Source: CAD feature listing. Evaluate the final solid. Frame: model axes, mm. A direction names the side the tool comes from. Round coordinates to 2 decimals unless told otherwise and drop trailing zeros. Order: outer loops, then holes, each group sorted by start corner. A loop starts at its lowest first (then second) coordinate and runs counter-clockwise, first axis right, second up. Notation, with made-up numbers: M -4,0.25 L 20,0.25 A28 ccw 20,28.25 Z; hole C 82.5,-3.5 d4. An arc over 180 degrees is marked long. Use one line per item in the form item = value. Start each with the question number.
Q1. Material intervals for probe 1 along X at (y, z) = (2.1, 39); probe 2 along Z at (x, y) = (1, 2.95); probe 3 along X at (y, z) = (1.6, -55), sorted ascending.
Q2. Pull-direction query (Z, two-part tool) for faces 1 (the conical face through (-41.21, 2.92, 39.85)), 2 (the conical face through (-41.21, 2.92, -37.93)), 3 (the flat face through (34, 5, -44)); classes: pulls with the +Z half, pulls with the -Z half, needs draft (parallel to the pull), parting line crosses it, or undercut.
Q3. Section A-A (z = -26). Return the cut outline in (x, y), plus the area to 3 significant figures.
Q4. Contact query for flat-ended pins moving along their axis: pin 1 (6 mm diameter, centred on x = -38.89, z = 38.89, fed in from +Y); pin 2 (5.5 mm diameter, centred on x = 55, z = 0, fed in from +Y). Output: stop coordinate, or through.
Q5. Section B-B (y = 1.3). Give the number of separate pieces and of enclosed holes in the cut face, plus the area to 3 significant figures.
Q6. Reachability of faces 4 (the flat face through (-39, 0, -1)), 5 (the cylindrical face through (-17.235, 4.507, 41.569)) from +Z, -Z, +X, -X, +Y, -Y: full face, straight path, thin tool, end or side. Return the list, or none.
from build123d import *

# Parameters (mm, degrees)
SKETCH1_W                                            = 327
SKETCH1_H                                            = 192
BOSS_EXTRUDE1_DEPTH                                  = 5
SKETCH2_R                                            = 35
CUT_EXTRUDE1_DEPTH                                   = 190.666154071
SKETCH3_R                                            = 45
CUT_EXTRUDE2_DEPTH                                   = 1
CSK_FOR_M4_HEX_SOCKET_COUNTERSUNK_HEAD_S_D           = 4.8
CSK_FOR_M4_HEX_SOCKET_COUNTERSUNK_HEAD_S_CSINK_D     = 9.18
CSK_FOR_M4_HEX_SOCKET_COUNTERSUNK_HEAD_S_CSINK_ANGLE = 90


with BuildPart() as part:
    # Sketch1 → Boss-Extrude1 (new body)
    with BuildSketch(Plane(origin=(0, 0, 0), x_dir=(1, 0, 0), z_dir=(0, 1, 0))):
        Rectangle(SKETCH1_W, SKETCH1_H)
    extrude(amount=BOSS_EXTRUDE1_DEPTH)

    # Sketch2 → Cut-Extrude1 (cut, through all)
    with BuildSketch(Plane(origin=(0, 5, 0), x_dir=(1, 0, 0), z_dir=(0, 1, 0))):
        with Locations(Location((0, 0, 0), (0, 0, 270))):
            Circle(SKETCH2_R)
    extrude(amount=-CUT_EXTRUDE1_DEPTH, mode=Mode.SUBTRACT)

    # Sketch3 → Cut-Extrude2 (cut)
    with BuildSketch(Plane(origin=(0, 5, 0), x_dir=(1, 0, 0), z_dir=(0, 1, 0))):
        with Locations(Location((0, 0, 0), (0, 0, 270))):
            Circle(SKETCH3_R)
    extrude(amount=-CUT_EXTRUDE2_DEPTH, mode=Mode.SUBTRACT)

    # CSK for M4 Hex Socket Countersunk Head Screw1 (through all)
    with Locations(Plane(origin=(0, 5, 0), x_dir=(1, 0, 0), z_dir=(0, 1, 0))):
        with Locations((-38.890872965, -38.890872965), (-55, 0), (-38.890872965, 38.890872965), (0, 55), (38.890872965, 38.890872965), (55, 0), (38.890872965, -38.890872965), (0, -55)):
            CounterSinkHole(CSK_FOR_M4_HEX_SOCKET_COUNTERSUNK_HEAD_S_D / 2, CSK_FOR_M4_HEX_SOCKET_COUNTERSUNK_HEAD_S_CSINK_D / 2, counter_sink_angle=CSK_FOR_M4_HEX_SOCKET_COUNTERSUNK_HEAD_S_CSINK_ANGLE)


solid = part.part
Results list:
q1.probe_1 = -163.5 to -41.29, -36.49 to 36.49, 41.29 to 163.5
q1.probe_2 = -96 to -57.33, -52.67 to -34.99, 34.99 to 52.67, 57.33 to 96
q1.probe_3 = -163.5 to -2.4, 2.4 to 163.5
q2.face_1 = undercut
q2.face_2 = undercut
q2.face_3 = needs draft
q3.outline = M -163.5,0 L -23.43,0 L -23.43,4 L -36.73,4 L -36.73,5 L -163.5,5 Z; M 23.43,0 L 163.5,0 L 163.5,5 L 36.73,5 L 36.73,4 L 23.43,4 Z
q3.area = 1,370 mm2
q4.pin_1 = 3.41
q4.pin_2 = 3.16
q5.separate_pieces = 1
q5.enclosed_holes = 9
q5.area = 58,800 mm2
q6.face_4 = +Z, -Z, +X, -X, -Y
q6.face_5 = +Y
